from build123d import *

# Parameters (mm, degrees)
SKETCH1_W           = 210
SKETCH1_H           = 116
SKETCH1_R           = 2.65
SKETCH1_R_2         = 11.25
SKETCH1_R_3         = 1.75
SKETCH1_R_4         = 2.6
BOSS_EXTRUDE1_DEPTH = 6
SKETCH4_R           = 1.25
CUT_EXTRUDE1_DEPTH  = 5.5
BOSS_EXTRUDE3_DEPTH = 1
BOSS_EXTRUDE4_DEPTH = 1
SKETCH4_5_R         = 1.25
CUT_EXTRUDE2_DEPTH  = 5.5
SKETCH6_W           = 80
SKETCH6_H           = 1
BOSS_EXTRUDE5_DEPTH = 3
FILLET1_R           = 0.5


with BuildPart() as part:
    # Sketch1 → Boss-Extrude1 (new body)
    with BuildSketch(Plane(origin=(0, 0, 0), x_dir=(1, 0, 0), z_dir=(0, 1, 0))):
        Rectangle(SKETCH1_W, SKETCH1_H)
        with Locations(Location((-95, 48, 0), (0, 0, 270))):
            Circle(SKETCH1_R, mode=Mode.SUBTRACT)
        with Locations(Location((95, 48, 0), (0, 0, 90))):
            Circle(SKETCH1_R, mode=Mode.SUBTRACT)
        with Locations(Location((95, -48, 0), (0, 0, 270))):
            Circle(SKETCH1_R, mode=Mode.SUBTRACT)
        with Locations(Location((-95, -48, 0), (0, 0, 90))):
            Circle(SKETCH1_R, mode=Mode.SUBTRACT)
        with Locations(Location((78, 6.11, 0), (0, 0, 270))):
            Circle(SKETCH1_R_2, mode=Mode.SUBTRACT)
        with Locations(Location((93.5, 21.61, 0), (0, 0, 270))):
            Circle(SKETCH1_R_3, mode=Mode.SUBTRACT)
        with Locations(Location((62.5, 21.61, 0), (0, 0, 270))):
            Circle(SKETCH1_R_3, mode=Mode.SUBTRACT)
        with Locations(Location((62.5, -9.39, 0), (0, 0, 270))):
            Circle(SKETCH1_R_3, mode=Mode.SUBTRACT)
        with Locations(Location((93.5, -9.39, 0), (0, 0, 270))):
            Circle(SKETCH1_R_3, mode=Mode.SUBTRACT)
        with Locations(Location((-90, -7, 0), (0, 0, 270))):
            Circle(SKETCH1_R_4, mode=Mode.SUBTRACT)
        with Locations(Location((0, 48, 0), (0, 0, 270))):
            Circle(SKETCH1_R, mode=Mode.SUBTRACT)
        with Locations(Location((0, -48, 0), (0, 0, 90))):
            Circle(SKETCH1_R, mode=Mode.SUBTRACT)
    extrude(amount=BOSS_EXTRUDE1_DEPTH)

    # Sketch4 → Cut-Extrude1 (cut)
    with BuildSketch(Plane(origin=(0, 6, 0), x_dir=(1, 0, 0), z_dir=(0, 1, 0))):
        with Locations(Location((49.9, 31.5, 0), (0, 0, 270))):
            Circle(SKETCH4_R)
        with Locations(Location((49.9, 22, 0), (0, 0, 270))):
            Circle(SKETCH4_R)
    extrude(amount=-CUT_EXTRUDE1_DEPTH, mode=Mode.SUBTRACT)

    # Sketch4<3> → Boss-Extrude3 (add)
    with BuildSketch(Plane(origin=(0, 6, 0), x_dir=(1, 0, 0), z_dir=(0, 1, 0))):
        Polygon((40.9, 37), (52.5, 37), (52.5, 16.7), (40.9, 16.7), (40.9, 14.7), (54.5, 14.7), (54.5, 38), (40.9, 38), align=None)
    extrude(amount=BOSS_EXTRUDE3_DEPTH)

    # Sketch4<4> → Boss-Extrude4 (add)
    with BuildSketch(Plane(origin=(0, 6, 0), x_dir=(1, 0, 0), z_dir=(0, 1, 0))):
        Polygon((-45, -16.7), (-33.4, -16.7), (-33.4, -14.7), (-47, -14.7), (-47, -38), (-33.4, -38), (-33.4, -37), (-45, -37), align=None)
    extrude(amount=BOSS_EXTRUDE4_DEPTH)

    # Sketch4<5> → Cut-Extrude2 (cut)
    with BuildSketch(Plane(origin=(0, 6, 0), x_dir=(1, 0, 0), z_dir=(0, 1, 0))):
        with Locations(Location((-42.4, -22, 0), (0, 0, 270))):
            Circle(SKETCH4_5_R)
        with Locations(Location((-42.4, -31.5, 0), (0, 0, 270))):
            Circle(SKETCH4_5_R)
    extrude(amount=-CUT_EXTRUDE2_DEPTH, mode=Mode.SUBTRACT)

    # Sketch6 → Boss-Extrude5 (add)
    with BuildSketch(Plane(origin=(0, 6, 0), x_dir=(1, 0, 0), z_dir=(0, 1, 0))):
        with Locations((0, 2.5)):
            Rectangle(SKETCH6_W, SKETCH6_H)
        with Locations((0, -4.5)):
            Rectangle(SKETCH6_W, SKETCH6_H)
    extrude(amount=BOSS_EXTRUDE5_DEPTH)

    # Fillet1
    fillet1_edges = [part.edges().sort_by_distance(p)[0] for p in [
        (54.5, 6, -26.35),
        (40, 6, -2.5),
        (40, 6, 4.5),
        (0, 6, -2),
        (0, 6, -3),
        (-40, 6, -2.5),
        (0, 6, 4),
        (-40, 6, 4.5),
        (0, 6, 5),
        (-47, 6, 26.35),
        (47.7, 6, -38),
        (47.7, 6, -14.7),
        (-40.2, 6, 14.7),
        (-40.2, 7, 38),
    ]]
    fillet(fillet1_edges, radius=FILLET1_R - 0.0001)  # a hair under: the kernel refuses the full size


solid = part.part
Can you work these out from the model? Positions are in its coordinate system, mm. A direction names the side the tool comes from. Round coordinates to 2 decimals unless told otherwise and drop trailing zeros. Order: outer loops, then holes, each group sorted by start corner. A loop starts at its lowest first (then second) coordinate and runs counter-clockwise, first axis right, second up. Notation, with made-up numbers: M 50.5,54 L 109.5,54 A21 ccw 109.5,68 Z; hole C -16,13.5 d10. An arc over 180 degrees is marked long. Use a Markdown table: item, result.
1) Imagine slicing it at B-B (x = -90). List the corners of the cut face in (y, z) for me, then the cut area to 3 significant figures.
Geometry says:
| item | result |
|---|---|
| outline | M 0,-58 L 6,-58 L 6,4.4 L 0,4.4 Z; M 0,9.6 L 6,9.6 L 6,58 L 0,58 Z |
| area | 665 mm² |
2) I'm going to push flat-ended pins straight in: P1, Ø1.1, axis at y = 8, z = -2.5, coming from the +X side; P2, Ø3, axis at x = 49.9, z = -31.5, coming from the +Y side; P3, Ø0.5, axis at y = 6.5, z = -22.5, coming from the -X side. Where does each tip first touch, or does it pass through?
Geometry says:
| item | result |
|---|---|
| P1 | stops at x = 40 |
| P2 | stops at y = 6 |
| P3 | stops at x = 52.5 |
3) Imagine slicing it at A-A (y = 3.75). Give the number of separate pieces and of enclosed holes in the cut face, then the cut area to 3 significant figures.
Geometry says:
| item | result |
|---|---|
| separate pieces | 1 |
| enclosed holes | 16 |
| area | 23,800 mm² |
4) Imagine slicing it at C-C (z = -11). List the corners of the cut face in (x, y) for me.
Geometry says:
| item | result |
|---|---|
| outline | M -105,0 L 67.87,0 L 67.87,6 L -105,6 Z; M 88.13,0 L 105,0 L 105,6 L 88.13,6 Z |
5) If I drill on line 1 along X through (y, z) = (2.8, -48); line 2 along X through (y, z) = (3.05, 7); line 3 along Z through (x, y) = (15, 7.5), over which ranges is the centre line in solid material (lowest first)?
Geometry says:
| item | result |
|---|---|
| line 1 | x = -105 to -97.65, -92.35 to -2.65, 2.65 to 92.35, 97.65 to 105 |
| line 2 | x = -105 to -92.6, -87.4 to 105 |
| line 3 | z = -3 to -2, 4 to 5 |
6) Imagine slicing it at D-D (x = -30). List the corners of the cut face in (y, z) for me, then the cut area to 3 significant figures.
Geometry says:
| item | result |
|---|---|
| outline | M 0,-58 L 6,-58 L 6,-3.5 A0.5 cw 6.5,-3 L 9,-3 L 9,-2 L 6.5,-2 A0.5 cw 6,-1.5 L 6,3.5 A0.5 cw 6.5,4 L 9,4 L 9,5 L 6.5,5 A0.5 cw 6,5.5 L 6,58 L 0,58 Z |
| area | 702 mm² |
7) If we mould it in two halves opening along Z, with no side actions, what happens to faces 1 (the face through (-0.117, 2.958, 50.647)), 2 (the face through (0.117, 2.958, -50.647)), 3 (the face through (-105, 3, 1)), 4 (the face through (-1, 3, 58))? For each: +Z half, -Z half, draft (parallel to the pull), parting line (faces both ways), or undercut.
Geometry says:
| item | result |
|---|---|
| face 1 | undercut |
| face 2 | undercut |
| face 3 | draft |
| face 4 | +Z half |
8) On a 3-axis mill with a long thin cutter (end or side, diameter ignored), from which of +Z, -Z, +X, -X, +Y, -Y can I reach the whole of each face in a straight line? I mean faces 5 (the face through (-97.59, 2.96, -48.57)), 6 (the face through (-45.3, 7, 24.4)). Say none if no direction works.
Geometry says:
| item | result |
|---|---|
| face 5 | +Y, -Y |
| face 6 | +Z, +X, -X, +Y |
